Verification items for this drawing (mm, ordinates from the low corner). A direction names the side the tool comes from. Coordinates: 2 decimals unless noted, no trailing zeros. Order: outer loops, then holes, each group sorted by start corner. A loop starts at its lowest first (then second) coordinate and runs counter-clockwise, first axis right, second up. Notation, with made-up numbers: M -14,35.25 L 9,35.25 A17 ccw 9,49.25 Z; hole C 21,-20 d3. An arc over 180 degrees is marked long. Return JSON: item names as keys, results as strings. Group by question number.
1. Section check C-C, the plane z = 8.5. Record the cut outline in (x, y).
2. Gauge pin test, flat ends, axial feed: pin 1 (2 mm diameter, centred on y = 1, z = 3, fed in from -X) (1 decimal); pin 2 (3 mm diameter, centred on y = 4, z = 7.5, fed in from +X); pin 3 (5 mm diameter, centred on x = 12.5, z = 12.5, fed in from -Y); pin 4 (1.2 mm diameter, centred on y = 2, z = 5, fed in from -X). Record the tip position at first contact, or that the pin passes through.
3. Section check D-D, the plane y = 4.5. Give the number of separate pieces and of enclosed holes in the cut face, plus the area to 3 significant figures.
4. Mould release check, pull along Z, two halves, no side actions. Record for the marked faces 4, 5 and 6: +Z half, -Z half, draft (parallel to the pull), parting line (faces both ways), or undercut.
5. Material ranges on line 1 along X through (y, z) = (2.25, 10.5) (1 decimal); line 2 along X through (y, z) = (1.9, 8.5); line 3 along Z through (x, y) = (7.25, 4) (1 decimal), recorded low to high.
6. Set-up check for the marked faces 1, 2 and 3: record each of +Z, -Z, +X, -X, +Y, -Y from which the full face is reachable in a straight line by a thin tool's end or side.
7. Section check A-A, the plane x = 12.5. Record the cut outline in (y, z) (3 decimals), plus the area to 3 significant figures.
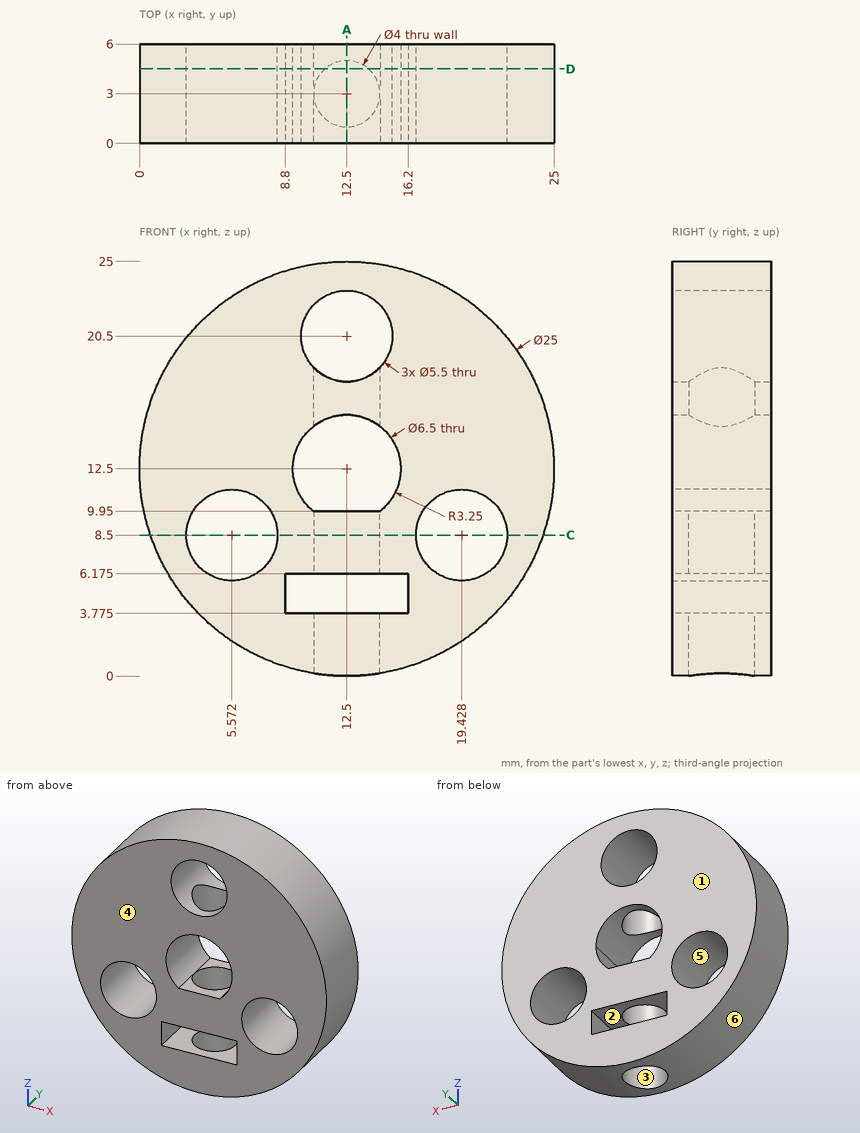
Answers follow:
{
 "1": {"outline": "M 0.66,0 L 2.82,0 L 2.82,6 L 0.66,6 Z; M 8.32,0 L 16.68,0 L 16.68,6 L 8.32,6 Z; M 22.18,0 L 24.34,0 L 24.34,6 L 22.18,6 Z; hole C 12.5,3 d4"},
 "2": {"pin 1": "x = 3.3", "pin 2": "x = 24.5", "pin 3": "through", "pin 4": "x = 2.08"},
 "3": {"separate pieces": "1", "enclosed holes": "2", "area": "345 mm^2"},
 "4": {"face 4": "draft", "face 5": "undercut", "face 6": "parting line"},
 "5": {"line 1": "0.2 to 3.7, 7.5 to 9.9, 15.1 to 17.5, 21.3 to 24.8", "line 2": "0.66 to 2.82, 8.32 to 10.83, 14.17 to 16.68, 22.18 to 24.34", "line 3": "1.2 to 6.3, 10.7 to 23.8"},
 "6": {"face 1": "+Z, -Z, +X, -X, +Y", "face 2": "+Y, -Y", "face 3": "-Z"},
 "7": {"outline": "M 0,0 L 1,0 L 1,3.775 L 0,3.775 Z; M 0,6.175 L 1,6.175 L 1,9.95 L 0,9.95 Z; M 0,15.75 L 1,15.75 L 1,17.75 L 0,17.75 Z; M 0,23.25 L 6,23.25 L 6,25 L 0,25 Z; M 5,0 L 6,0 L 6,3.775 L 5,3.775 Z; M 5,6.175 L 6,6.175 L 6,9.95 L 5,9.95 Z; M 5,15.75 L 6,15.75 L 6,17.75 L 5,17.75 Z", "area": "29.6 mm^2"}
}
